For this review, use the dimensioned drawing (mm, ordinates from the lowest corner) and the shaded views. A direction names the side the tool comes from. Coordinates: 2 decimals unless noted, no trailing zeros. Loops run counter-clockwise (first coordinate to the right, second up) from the corner with the lowest first, then second, coordinate; pieces in that order, holes last. Notation, with made-up numbers: (-20, -35.5) - (21, -35.5) arc R32 cw to (21, -1.5) - close; hole circle Ø4 at (70, 79.5). An arc over 180 degrees is marked (long way). Answer in a Markdown table with one row per item. Add a question column.
(1) The part is to be moulded in two halves that separate along Y. For the marked faces 4, 5 and 6, say which applies: released by +Y, released by -Y, zero draft, split by the parting line, or undercut.
(2) Clearance check with flat-ended pins moving along their axes: pin 1 (9 mm diameter, centred on x = 27.5, z = 75, fed in from -Y); pin 2 (15 mm diameter, centred on y = 113.5, z = 39.5, fed in from +X); pin 3 (6.5 mm diameter, centred on x = 62.5, y = 101.5, fed in from -Z); pin 4 (1.5 mm diameter, centred on x = 48.5, z = 30.5, fed in from -Y). State where each tip first meets the part, or that it passes through.
(3) For the marked faces 1, 2 and 3, list the 3-axis set-ups (+Z, -Z, +X, -X, +Y, -Y) from which the entire face can be reached by the end or side of a thin tool; tool diameter is ignored.
(4) We need section B-B, the plane z = 14. Write out the cut boundary in (x, y), plus the area to 3 significant figures.
(5) We need section A-A, the plane x = 30. Write out the cut boundary in (y, z).
(6) To check wall thickness, follow L1, parallel to Z at x = 76, y = 29.5; L2, parallel to Y at x = 37, z = 69; L3, parallel to X at y = 101, z = 69.5. State the ranges of each line that lie inside material, in increasing order. Write a range as [from, to].
(7) We need section D-D, the plane x = 82. Write out the cut boundary in (y, z).
(8) We need section C-C, the plane x = 55. Write out the cut boundary in (y, z).
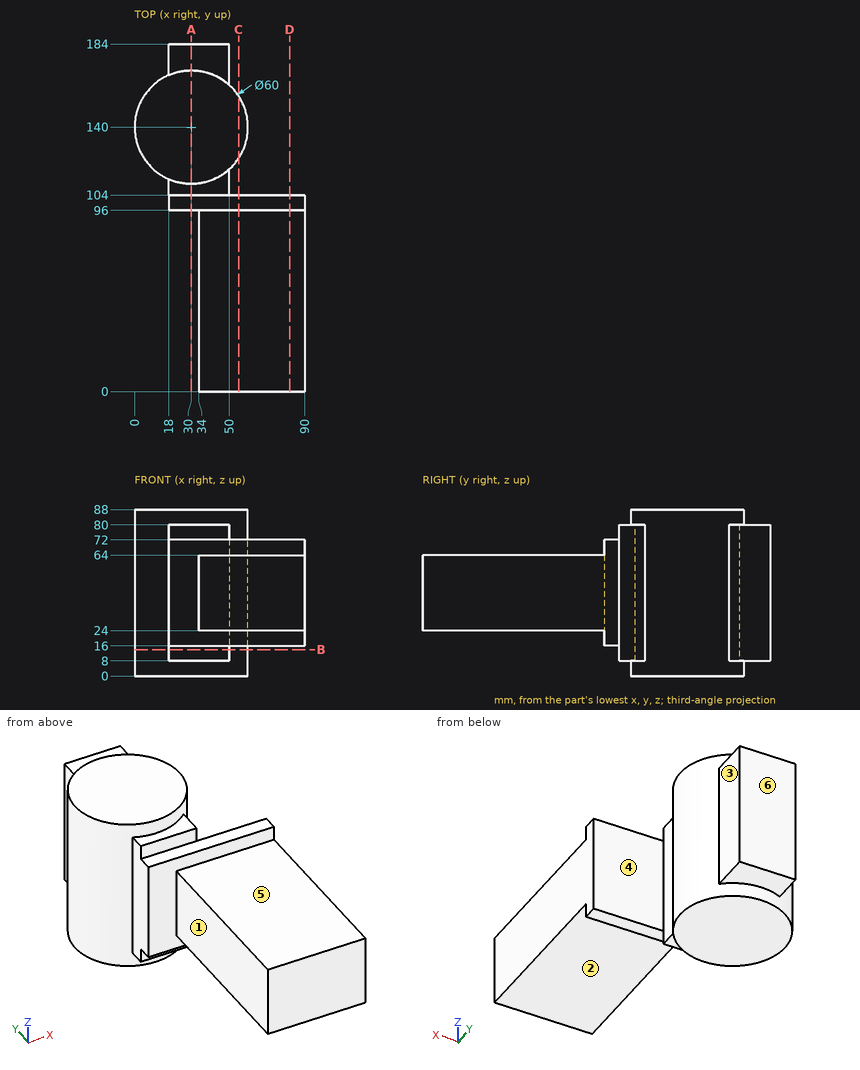
Responses:
| question | item | result |
|---|---|---|
| 1 | face 4 | undercut |
| 1 | face 5 | zero draft |
| 1 | face 6 | released by +Y |
| 2 | pin 1 | stops at y = 96 |
| 2 | pin 2 | stops at x = 53.22 |
| 2 | pin 3 | stops at z = 16 |
| 2 | pin 4 | stops at y = 0 |
| 3 | face 1 | +Z, -Z, -X, -Y |
| 3 | face 2 | -Z, +X, -X, -Y |
| 3 | face 3 | +Z, -Z, +X, +Y |
| 4 | outline | (18, 104) - (50, 104) - (50, 117.64) arc R30 ccw to (50, 162.36) - (50, 184) - (18, 184) - (18, 167.5) arc R30 ccw to (18, 112.5) - close |
| 4 | area | 3,580 mm2 |
| 5 | outline | (96, 16) - (104, 16) - (104, 8) - (110, 8) - (110, 0) - (170, 0) - (170, 8) - (184, 8) - (184, 80) - (170, 80) - (170, 88) - (110, 88) - (110, 80) - (104, 80) - (104, 72) - (96, 72) - close |
| 6 | L1 | z = [24, 64] |
| 6 | L2 | y = [96, 184] |
| 6 | L3 | x = [18, 90] |
| 7 | outline | (0, 24) - (96, 24) - (96, 16) - (104, 16) - (104, 72) - (96, 72) - (96, 64) - (0, 64) - close |
| 8 | outline | (0, 24) - (96, 24) - (96, 16) - (104, 16) - (104, 72) - (96, 72) - (96, 64) - (0, 64) - close; (123.42, 0) - (156.58, 0) - (156.58, 88) - (123.42, 88) - close |
